For this review, use the dimensioned drawing (mm, ordinates from the lowest corner) and the shaded views. Round coordinates to 2 decimals unless told otherwise and drop trailing zeros. Write each loop counter-clockwise with the first axis right and the second up, starting at its lowest first coordinate (ties: lowest second). Pieces come first, ordered by that corner, then holes. Notation, with made-up numbers: M -27.75,74.25 L -21.75,74.25 A23 ccw -21.75,103.25 Z; hole C 4.25,78 d11. An arc over 180 degrees is marked long. One line per question, with ' | ' between items.
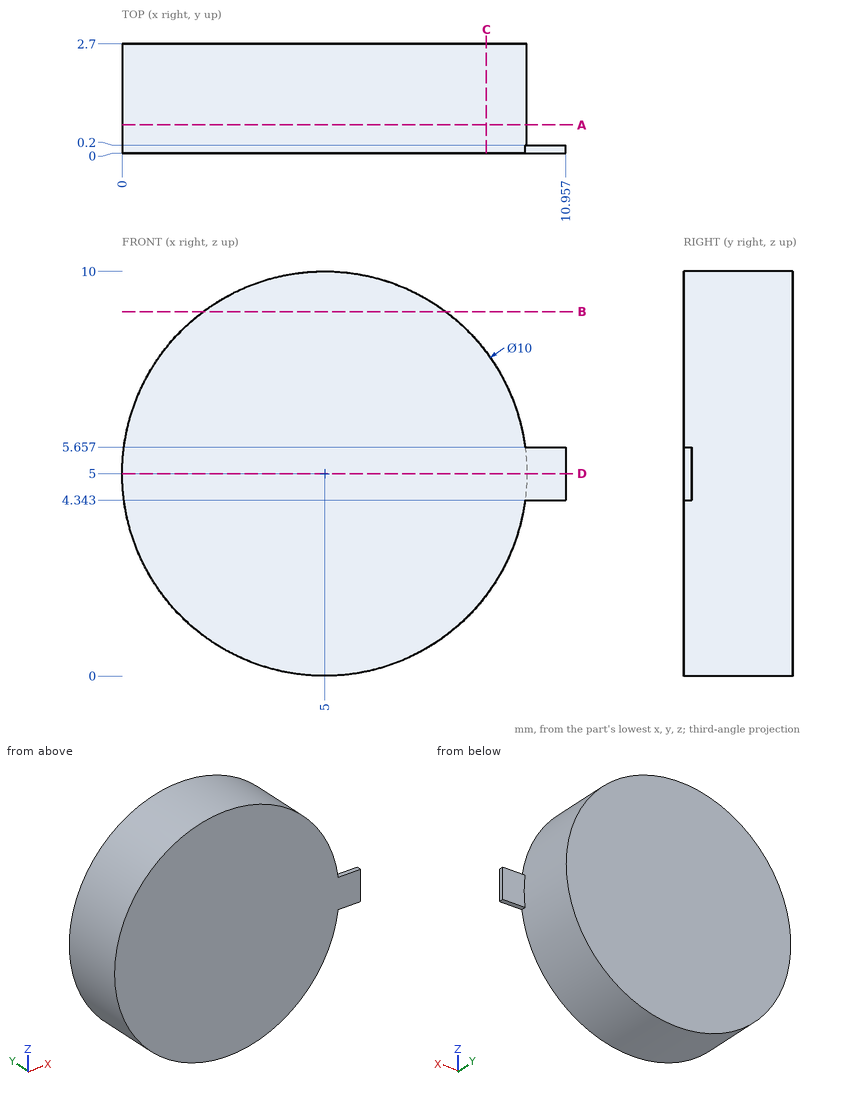
Item 1: To check wall thickness, follow line 1 along X through (y, z) = (1.75, 7); line 2 along Z through (x, y) = (2.5, 2.45); line 3 along X through (y, z) = (0.65, 1.75). State the ranges of each line that lie inside material, in increasing order. Write a range as from..to.
Results:
line 1: 0.42..9.58 | line 2: 0.67..9.33 | line 3: 1.2..8.8
Item 2: Take a section at C-C (x = 9). Write out the cut boundary in (y, z).
Results:
outline: M 0,2 L 2.7,2 L 2.7,8 L 0,8 Z
Item 3: Take a section at A-A (y = 0.7). Write out the cut boundary in (x, z).
Results:
outline: C 5,5 d10
Item 4: Take a section at B-B (z = 9). Write out the cut boundary in (x, y).
Results:
outline: M 2,0 L 8,0 L 8,2.7 L 2,2.7 Z
Item 5: Take a section at D-D (z = 5). Write out the cut boundary in (x, y), then the cut area to 3 significant figures.
Results:
outline: M 0,0 L 10.96,0 L 10.96,0.2 L 10,0.2 L 10,2.7 L 0,2.7 Z | area: 27.2 mm2
Item 6: Insertion check: pin 1 Ø0.8 at (x, z) = (10.5, 5) entering from +Y; pin 2 Ø1.5 at (y, z) = (2, 7) entering from -X. Each pin has a flat end and moves straight along its axis. Give the tip position at first contact, or say it passes through.
Results:
pin 1: y = 0.2 | pin 2: x = 0.16
